```python
from build123d import *

# Parameters (mm, degrees)
SKETCH1_W           = 46
SKETCH1_H           = 36
BOSS_EXTRUDE1_DEPTH = 15
BOSS_EXTRUDE2_DEPTH = 3
SKETCH3_R           = 7.75
CUT_EXTRUDE1_DEPTH  = 10
SKETCH4_W           = 5
SKETCH4_H           = 5
SKETCH4_R           = 1
BOSS_EXTRUDE3_DEPTH = 10
FILLET1_R           = 2.5
SKETCH6_R           = 1
CUT_EXTRUDE2_DEPTH  = 10
CHAMFER1_SIZE       = 2
FILLET2_R           = 2
SKETCH7_W           = 13
SKETCH7_H           = 4.5
CUT_EXTRUDE3_DEPTH  = 10
SKETCH8_W           = 9
SKETCH8_H           = 4
CUT_EXTRUDE4_DEPTH  = 10
SKETCH9_W           = 2
SKETCH9_H           = 4
CUT_EXTRUDE5_DEPTH  = 10


with BuildPart() as part:
    # Sketch1 → Boss-Extrude1 (new body)
    with BuildSketch(Plane.XY):
        Polygon((-15, -27.5), (-15, -20), (25, -20), (25, 20), (5, 20), (5, 27.5), (-25, 27.5), (-25, -27.5), align=None)
        Rectangle(SKETCH1_W, SKETCH1_H, mode=Mode.SUBTRACT)
    extrude(amount=BOSS_EXTRUDE1_DEPTH)

    # Sketch2 → Boss-Extrude2 (add)
    with BuildSketch(Plane.XY.offset(15)):
        Polygon((-25, 27.5), (-25, -27.5), (-15, -27.5), (-15, -20), (25, -20), (25, 20), (5, 20), (5, 27.5), align=None)
    extrude(amount=BOSS_EXTRUDE2_DEPTH)

    # Sketch3 → Cut-Extrude1 (cut)
    with BuildSketch(Plane.XY.offset(18)):
        with Locations((-10.25, 0)):
            Circle(SKETCH3_R)
    extrude(amount=-CUT_EXTRUDE1_DEPTH, mode=Mode.SUBTRACT)

    # Sketch4 → Boss-Extrude3 (add)
    # profile 1 of 4: a face of its own
    with BuildSketch(Plane(origin=(0, 0, 15), x_dir=(-1, 0, 0), z_dir=(0, 0, -1))):
        with Locations((20.5, -15.5)):
            Rectangle(SKETCH4_W, SKETCH4_H)
        with Locations((20.252039878, -15.196246514)):
            Circle(SKETCH4_R, mode=Mode.SUBTRACT)
    # profile 2 of 4: a face of its own
    with BuildSketch(Plane(origin=(0, 0, 15), x_dir=(-1, 0, 0), z_dir=(0, 0, -1))):
        with Locations((-3.747960122, -15.5)):
            Rectangle(SKETCH4_W, SKETCH4_H)
        with Locations((-3.747960122, -15.196246514)):
            Circle(SKETCH4_R, mode=Mode.SUBTRACT)
    # profile 3 of 4: a face of its own
    with BuildSketch(Plane(origin=(0, 0, 15), x_dir=(-1, 0, 0), z_dir=(0, 0, -1))):
        with Locations((-3.747960122, 15.5)):
            Rectangle(SKETCH4_W, SKETCH4_H)
        with Locations((-3.747960122, 15.203753486)):
            Circle(SKETCH4_R, mode=Mode.SUBTRACT)
    # profile 4 of 4: a face of its own
    with BuildSketch(Plane(origin=(0, 0, 15), x_dir=(-1, 0, 0), z_dir=(0, 0, -1))):
        with Locations((20.5, 15.5)):
            Rectangle(SKETCH4_W, SKETCH4_H)
        with Locations((20.252039878, 15.203753486)):
            Circle(SKETCH4_R, mode=Mode.SUBTRACT)
    extrude(amount=BOSS_EXTRUDE3_DEPTH)

    # Fillet1
    fillet1_edges = [part.edges().sort_by_distance(p)[0] for p in [
        (1.247960122, 13, 10),
        (6.247960122, 13, 10),
        (-18, 13, 10),
        (-18, -13, 10),
        (1.247960122, -13, 10),
        (6.247960122, -13, 10),
    ]]
    fillet(fillet1_edges, radius=FILLET1_R - 0.0001)  # a hair under: the kernel refuses the full size

    # Sketch6 → Cut-Extrude2 (cut)
    with BuildSketch(Plane(origin=(0, 0, -3), x_dir=(-1, 0, 0), z_dir=(0, 0, -1))):
        with Locations((0, 22.5)):
            Circle(SKETCH6_R)
        with Locations((20, 22.5)):
            Circle(SKETCH6_R)
        with Locations((20, -22.5)):
            Circle(SKETCH6_R)
    extrude(amount=-CUT_EXTRUDE2_DEPTH, mode=Mode.SUBTRACT)

    # Chamfer1
    chamfer1_edges = [part.edges().sort_by_distance(p)[0] for p in [
        (5, 27.5, 9),
        (5, 20, 9),
        (-15, -20, 9),
        (-15, -27.5, 9),
    ]]
    chamfer(chamfer1_edges, length=CHAMFER1_SIZE)

    # Fillet2
    fillet2_edges = [part.edges().sort_by_distance(p)[0] for p in [
        (-25, 27.5, 9),
        (25, 20, 9),
        (25, -20, 9),
        (-25, -27.5, 9),
    ]]
    fillet(fillet2_edges, radius=FILLET2_R)

    # Sketch7 → Cut-Extrude3 (cut)
    with BuildSketch(Plane.XZ.offset(-18)):
        with Locations((13.2, 2.25)):
            Rectangle(SKETCH7_W, SKETCH7_H)
    extrude(amount=-CUT_EXTRUDE3_DEPTH, mode=Mode.SUBTRACT)

    # Sketch8 → Cut-Extrude4 (cut)
    with BuildSketch(Plane(origin=(0, -18, 0), x_dir=(1, 0, 0), z_dir=(0, 1, 0))):
        Polygon((22.2, 0), (9.2, 0), (9.2, -4.5), (11.7, -4.5), (11.7, -9.5), (22.2, -9.5), align=None)
        with Locations((-3.8, -6.2)):
            Rectangle(SKETCH8_W, SKETCH8_H)
    extrude(amount=-CUT_EXTRUDE4_DEPTH, mode=Mode.SUBTRACT)

    # Sketch9 → Cut-Extrude5 (cut)
    with BuildSketch(Plane.ZY.offset(-23)):
        with Locations((5.65, 14.2)):
            Rectangle(SKETCH9_W, SKETCH9_H)
    extrude(amount=-CUT_EXTRUDE5_DEPTH, mode=Mode.SUBTRACT)


solid = part.part
```
Model file for the job. Use its own axes, mm. A direction names the side the tool comes from. Coordinates: 2 decimals unless noted, no trailing zeros. Loops run counter-clockwise (first coordinate to the right, second up) from the corner with the lowest first, then second, coordinate; pieces in that order, holes last. Notation, with made-up numbers: (42.25, -19.5) - (71.25, -19.5) arc R13 ccw to (71.25, -2.5) - close; hole circle Ø8 at (67.25, 12.25). An arc over 180 degrees is marked (long way). Write item = value, one per line. Start each with the question number.
Item 1: Saw through at A-A, the plane z = 2.75. State how many separate pieces and enclosed holes the cut face has, then the cut area to 3 significant figures.
Item 2: Pull direction Y, two halves, no side cores. Call faces 1 (the face through (24, 14, 6.65)), 2 (the face through (0, 0, 18)), 3 (the face through (-21, 16.1, 5)), 4 (the face through (-24.43, 26.9, 8.87)): +Y half, -Y half, draft (parallel to the pull), parting line (faces both ways), or undercut.
Item 3: Saw through at D-D, the plane y = -11. List the corners of the cut face in (x, z), then the cut area to 3 significant figures.
Item 4: Saw through at C-C, the plane y = 0. List the corners of the cut face in (x, z).
Item 5: Saw through at B-B, the plane x = -10.25. List the corners of the cut face in (y, z).
Item 6: 3-axis set-ups, long thin cutter, end or side, ignore diameter. For faces 5 (the face through (13, 19, 4.5)), 6 (the face through (-18.713, -13.752, 9.93)), 7 (the face through (5, 24, 9)), 8 (the face through (-15, -24, 9)), 9 (the face through (24, 12.2, 6)): which of +Z, -Z, +X, -X, +Y, -Y reach the whole face in a straight line?
Item 7: Wall check: probe 1 along Y at (x, z) = (-10.25, 16.75); probe 2 along X at (y, z) = (-12, 2.75); probe 3 along Y at (x, z) = (-11, 6.5). Give the ranges that are in metal, low to high. Write a range as [from, to].
Item 8: Drop flat-ended pins along their axis: pin 1 Ø5 at (x, y) = (-6.5, 10.5) entering from -Z; pin 2 Ø0.6 at (x, y) = (-20.5, 14.5) entering from -Z; pin 3 Ø2 at (x, y) = (12, 19) entering from -Z. Give the stop position or say it passes through.
Answers:
q1.separate_pieces = 2
q1.enclosed_holes = 3
q1.area = 579 mm2
q2.face_1 = undercut
q2.face_2 = draft
q2.face_3 = undercut
q2.face_4 = +Y half
q3.outline = (-25, 0) - (-23, 0) - (-23, 15) - (23, 15) - (23, 0) - (25, 0) - (25, 18) - (-25, 18) - close
q3.area = 210 mm2
q4.outline = (-25, 0) - (-23, 0) - (-23, 15) - (-18, 15) - (-18, 18) - (-25, 18) - close; (-2.5, 15) - (23, 15) - (23, 0) - (25, 0) - (25, 18) - (-2.5, 18) - close
q5.outline = (-20, 0) - (-18, 0) - (-18, 15) - (-7.75, 15) - (-7.75, 18) - (-20, 18) - close; (7.75, 15) - (18, 15) - (18, 0) - (27.5, 0) - (27.5, 18) - (7.75, 18) - close
q6.face_5 = -Z, +Y
q6.face_6 = -Z
q6.face_7 = +Z, -Z, +X, +Y
q6.face_8 = +Z, -Z, +X, -Y
q6.face_9 = +X
q7.probe_1 = [-20, -7.75], [7.75, 27.5]
q7.probe_2 = [-25, -23], [23, 25]
q7.probe_3 = [-20, -18], [18, 27.5]
q8.pin_1 = 15
q8.pin_2 = 5
q8.pin_3 = 4.5
